from build123d import *

# Parameters (mm, degrees)
EXTRUDE_START       = -3
EXTRUDE_1_DEPTH     = 8
EXTRUDE_2_DEPTH     = 8
CUT_EXTRUDE_1_DEPTH = 24.482669171


with BuildPart() as part:
    # 草图2 → 凸台-拉伸1 (new body)
    with BuildSketch(Plane.XY.offset(EXTRUDE_START)):
        with BuildLine():
            Line((0.452812855, -3.974287423), (50.958977377, 1.780163155))
            Line((50.958977377, 1.780163155), (60, 7))
            Line((60, 7), (60, 11))
            Line((60, 11), (54.92820323, 11))
            Line((54.92820323, 11), (49.039778636, 7.600316475))
            Line((49.039778636, 7.600316475), (17.440206483, 4))
            Line((17.440206483, 4), (0, 4))
            ThreePointArc((0, 4), (-3.993566682, -0.22677115), (0.452812855, -3.974287423))
        make_face()
    extrude(amount=-EXTRUDE_1_DEPTH)

    # 草图3 → 凸台-拉伸2 (add)
    with BuildSketch(Plane(origin=(0, 0, -11), x_dir=(-1, 0, 0), z_dir=(0, 0, -1))):
        Polygon((-27.201059955, -0.926709618), (-33.142680696, 5.789070951), (-49.039778636, 7.600316475), (-54.92820323, 11), (-60, 11), (-60, 7), (-50.958977377, 1.780163155), align=None)
    extrude(amount=EXTRUDE_2_DEPTH)

    # 草图4 → 切除-拉伸1 (cut, through all, along a direction that is not the sketch's normal)
    with BuildSketch(Plane(origin=(0.452812855, -3.974287423, 0), x_dir=(0.993571856, 0.113203214, 0), z_dir=(0.113203214, -0.993571856, 0))):
        Polygon((26.921301109, -11), (26.921301109, -19), (60.859546692, -19), align=None)
        Polygon((26.921301109, -3), (60.859546692, -15.352511196), (60.859546692, -3), align=None)
    extrude(amount=-CUT_EXTRUDE_1_DEPTH, dir=(-0.662620048, -0.748955721, 0), mode=Mode.SUBTRACT)


solid = part.part
Can you work these out from the model? Positions are in its coordinate system, mm. A direction names the side the tool comes from. Coordinates: 2 decimals unless noted, no trailing zeros. Loops run counter-clockwise (first coordinate to the right, second up) from the corner with the lowest first, then second, coordinate; pieces in that order, holes last. Notation, with made-up numbers: (64.25, -3) - (101.25, -3) arc R34 ccw to (101.25, 29) - close; hole circle Ø7 at (72.5, 40.5). An arc over 180 degrees is marked (long way). Put each result on its own line as item: value. Start each with the question number.
Item 1: For pin 1 (5 mm diameter, centred on x = 33.5, z = -11, fed in from -Y); pin 2 (8 mm diameter, centred on x = 43, y = 2.5, fed in from +Z); pin 3 (8 mm diameter, centred on x = 8, y = -1, fed in from -Z), each with a flat end and sliding along its axis, tell me the tip position at first contact or that it passes through.
Item 2: Suppose I cut it at A-A (z = -12.75). Please give me the cut outline in (x, y).
Item 3: Which directions (+Z, -Z, +X, -X, +Y, -Y) give clear straight access to the entire face, cutting with the end or side of a thin tool? Please do faces 1 (the face through (14, 1, -3)), 2 (the face through (9, 4, -7)).
Item 4: If I drill on line 1 along Z through (x, y) = (9, 3.25); line 2 along Y through (x, z) = (53, -15.25); line 3 along X through (y, z) = (2.5, -10.75), over which ranges is the centre line in solid material (lowest first)?
Item 5: Suppose I cut it at B-B (x = 39.5). Please give me the cut outline in (y, z), and give its area (3 significant figures).
Item 6: Suppose I cut it at C-C (y = 0). Please give me the cut outline in (x, z), and give its area (3 significant figures).
Item 7: Suppose I cut it at D-D (x = 46). Please give me the cut outline in (y, z), and give its area (3 significant figures).
Here are the results:
1. pin 1: y = -0.49
1. pin 2: z = -6.03
1. pin 3: z = -11
2. outline: (34.58, -0.09) - (50.96, 1.78) - (56.21, 4.81) - (60, 9.09) - (60, 11) - (54.93, 11) - (49.04, 7.6) - (40.52, 6.63) - close
3. face 1: +Z, +X, -X, +Y, -Y
3. face 2: +Z, -Z, -X, +Y
4. line 1: -11 to -3
4. line 2: 2.96 to 9.89
4. line 3: -3.12 to 49.26
5. outline: (0.47, -13.92) - (6.51, -12.51) - (6.51, -5.33) - (0.47, -7.51) - close
5. area: 41.0 mm²
6. outline: (-4, -11) - (28.02, -11) - (35.33, -12.93) - (35.33, -5.98) - (28.02, -3) - (-4, -3) - close
6. area: 311 mm²
7. outline: (1.22, -15.46) - (7.25, -14.05) - (7.25, -7.71) - (1.22, -9.89) - close
7. area: 36.0 mm²
